from build123d import *

# Parameters (mm, degrees)
F0_W     = 122.230552
F0_H     = 77.007032
F1_DEPTH = 30.48
F2_W     = 112.040394
F2_H     = 65.861254
F3_DEPTH = 120.65
F4_R     = 6.306585
F5_DEPTH = 227.33
F6_W     = 53.315248
F6_H     = 12.666776
F7_DEPTH = 179.578


with BuildPart() as f1:
    # F0 (on Top) → F1 (new body)
    with BuildSketch(Plane.XY):
        Rectangle(F0_W, F0_H)
    extrude(amount=F1_DEPTH)

    # F2 (on face) → F3 (cut)
    with BuildSketch(Plane(origin=(0, 0, 0), x_dir=(1, 0, 0), z_dir=(0, 0, -1))):
        Rectangle(F2_W, F2_H)
    extrude(amount=-F3_DEPTH, mode=Mode.SUBTRACT)

    # F4 (on face) → F5 (cut)
    with BuildSketch(Plane.YZ.offset(61.115276)):
        with Locations((0, 15.667252)):
            Circle(F4_R)
    extrude(amount=-F5_DEPTH, mode=Mode.SUBTRACT)

    # F6 (on face) → F7 (cut)
    with BuildSketch(Plane.XZ.offset(38.503516)):
        with Locations((0, 6.333388)):
            Rectangle(F6_W, F6_H)
    extrude(amount=-F7_DEPTH, mode=Mode.SUBTRACT)


solid = f1.part
Input: part model. Units: mm. Frame: model coordinates. A direction names the side the tool comes from. Give positions to 0.01 mm unless a question says otherwise; leave off trailing zeros. Order: outer loops, then holes, each group sorted by start corner. A loop starts at its lowest first (then second) coordinate and runs counter-clockwise, first axis right, second up. Notation, with made-up numbers: (-15.5, 71) -> (20.5, 71) arc R25 cw to (20.5, 89) -> close; hole circle Ø8 at (-20, 2.5). An arc over 180 degrees is marked (long way). Use one line per item in the form item = value.
1) Section D-D, the plane z = 24. Return loops of the section in (x, y).
Response values:
outline = (-61.12, -38.5) -> (61.12, -38.5) -> (61.12, 38.5) -> (-61.12, 38.5) -> close; hole (-56.02, -32.93) -> (56.02, -32.93) -> (56.02, 32.93) -> (-56.02, 32.93) -> close
2) Line query: probe 1 along X at (y, z) = (22.5, 26.5); probe 2 along Y at (x, z) = (-37.5, 23); probe 3 along Z at (x, y) = (-58, 0). Output: solid intervals per line, ascending.
Response values:
probe_1 = -61.12 to -56.02, 56.02 to 61.12
probe_2 = -38.5 to -32.93, 32.93 to 38.5
probe_3 = 0 to 9.36, 21.97 to 30.48
3) Mould query, pull axis Y, two halves, no side actions, for faces 1 (the cylindrical face through (58.6, -1.37, 9.51)), 2 (the flat face through (61.115, -1, 8)), 3 (the flat face through (-1, 38.504, 18)). Classes: pulls with the +Y half, pulls with the -Y half, needs draft (parallel to the pull), parting line crosses it, or undercut.
Response values:
face_1 = undercut
face_2 = needs draft
face_3 = pulls with the +Y half
4) Section C-C, the plane y = 0. Return loops of the section in (x, z), and give its area (3 significant figures).
Response values:
outline = (-61.12, 0) -> (-56.02, 0) -> (-56.02, 9.36) -> (-61.12, 9.36) -> close; (-61.12, 21.97) -> (-56.02, 21.97) -> (-56.02, 30.48) -> (-61.12, 30.48) -> close; (56.02, 0) -> (61.12, 0) -> (61.12, 9.36) -> (56.02, 9.36) -> close; (56.02, 21.97) -> (61.12, 21.97) -> (61.12, 30.48) -> (56.02, 30.48) -> close
area = 182 mm^2
5) Reachability of faces 4 (the flat face through (26.658, -36, 6)), 5 (the flat face through (-1, 32.931, 18)), 6 (the cylindrical face through (-58.53, -1.37, 9.51)) from +Z, -Z, +X, -X, +Y, -Y: full face, straight path, thin tool, end or side. Return the list, or none.
Response values:
face_4 = -Z, +Y, -Y
face_5 = +Z, -Z
face_6 = +X, -X
6) Section B-B, the plane x = -11.5. Return loops of the section in (y, z), and give its area (3 significant figures).
Response values:
outline = (-38.5, 12.67) -> (-32.93, 12.67) -> (-32.93, 30.48) -> (-38.5, 30.48) -> close; (32.93, 12.67) -> (38.5, 12.67) -> (38.5, 30.48) -> (32.93, 30.48) -> close
area = 199 mm^2
7) First-contact query: pin 1 Ø1.7 at (x, y) = (11.5, 34.5) entering from -Z. Flat tip, straight axial feed; report the tip coordinate or a pass-through.
Response values:
pin_1 = 12.67
8) Section A-A, the plane y = 10. Return loops of the section in (x, z), and give its area (3 significant figures).
Response values:
outline = (-61.12, 0) -> (-56.02, 0) -> (-56.02, 30.48) -> (-61.12, 30.48) -> close; (56.02, 0) -> (61.12, 0) -> (61.12, 30.48) -> (56.02, 30.48) -> close
area = 311 mm^2
